Autodesk Inventor part; units mm, degrees
ref_plane "YZ Plane" through (0, 0, 0) normal (1, 0, 0) x (0, 1, 0)
ref_plane "XZ Plane" through (0, 0, 0) normal (0, 1, 0) x (-1, 0, 0)
ref_plane "XY Plane" through (0, 0, 0) normal (0, 0, 1) x (1, 0, 0)
sketch "Sketch1" plane through (0, 0, 0) normal (0, 0, 1) x (1, 0, 0)
  line L0 (-168.2745, 480.6024) -> (-113.8232, 480.6024)
  line L1 (-73.2956, 353.1342) -> (-73.2956, 2.8452)
  line L2 (-73.2956, 2.8452) -> (-375.9641, 2.8452)
  line L3 (-375.9641, 2.8452) -> (-375.9641, 41.7492)
  arc A0 (-375.9641, 41.7492) -> (-168.2745, 480.6024) centre (-397.1456, 320.3452) ccw
  line L4 (-168.2745, 480.6024) -> (-245.12, 590.3492) construction
  line L5 (-245.12, 590.3492) -> (-245.12, 480.6024) construction
  line L6 (-245.12, 480.6024) -> (-168.2745, 480.6024) construction
  line L7 (-117.7456, 320.3452) -> (-117.7456, 124.3972) construction
  line L8 (-397.1456, 40.9452) -> (-554.9899, 40.9452) construction
  arc A1 (-73.2956, 353.1342) -> (-113.8232, 480.6024) centre (-397.1456, 320.3452) ccw
  dimension "d4" = 279.4
  dimension "d6" = 55
  dimension "d17" = 44.45
  dimension "d22" = 38.1
extrude "Extrusion1" add sketch "Sketch1" along normal blind 1.5875
sketch "Sketch2" plane through (0, 0, 1.5875) normal (0, 0, 1) x (1, 0, 0)
  arc A0 (-375.9641, 41.7492) -> (-168.2745, 480.6024) centre (-397.1456, 320.3452) ccw
  arc A1 (-375.9641, 41.7492) -> (-168.2745, 480.6024) centre (-397.1456, 320.3452) ccw
  arc A2 (-375.603, 37.0004) -> (-164.3733, 483.3341) centre (-397.1456, 320.3452) ccw
  line L0 (-397.1456, 320.3452) -> (-164.3733, 483.3341)
  line L1 (-168.2745, 480.6024) -> (-164.3733, 483.3341)
  line L2 (-397.1456, 320.3452) -> (-375.603, 37.0004)
  line L3 (-375.603, 37.0004) -> (-375.9641, 41.7492)
  point P0 (0, 0)
  dimension "d21" = 4.7625
extrude "Extrusion2" add sketch "Sketch2" along normal blind 15.875 and the other way blind 19.05 contours A0 L0 A2 L2
fillet "Fillet1" radius 25.4 1 edges at (-113.8232, 480.6024, 0.7937)
properties part number "ShooterCurve" material "Aluminum-6061"
The model under review builds one solid part; all positions refer to its coordinate system, in mm. Give positions to 0.01 mm unless a question says otherwise; leave off trailing zeros. Loops run counter-clockwise (first coordinate to the right, second up) from the corner with the lowest first, then second, coordinate; pieces in that order, holes last. Notation, with made-up numbers: (39, 37.5) -> (95, 37.5) arc R28 cw to (95, 68.5) -> close; hole circle Ø10 at (54, -7). An arc over 180 degrees is marked (long way). Put each result on its own line as item: value. Start each with the question number.
1. We need section A-A on x = -144. State the section outline as (y, z) points.
2. Clearance check with flat-ended pins moving along their axes: P1, Ø1.5, axis at x = -270, z = 12, coming from the -Y side; P2, Ø1.3, axis at x = -143, z = 0.5, coming from the +Y side; P3, Ø1.5, axis at x = -249.5, z = 2.5, coming from the +Y side. State where each tip first meets the part, or that it passes through.
3. We need section C-C on x = -347. State the section outline as (y, z) points, then the cut area to 3 significant figures.
4. We need section B-B on y = 416.5. State the section outline as (x, z) points, then the cut area to 3 significant figures.
5. Wall thickness on probe 1 along Z at (x, y) = (-139.5, 141.5); probe 2 along Y at (x, z) = (-149.5, 10); probe 3 along Y at (x, z) = (-155.5, 10): over which ranges is each line inside the solid? List them lowest first.
6. Mouldability with a two-part tool opening along Y and no side actions: class faces 1 (the face through (-142.865, 204.562, -0.244)), 2 (the face through (-147, 137, 1.588)), 3 (the face through (-84.865, 412.187, 0.783)) as released by +Y, released by -Y, zero draft, split by the parting line, or undercut.
7. We need section D-D on z = 12.5. State the section outline as (x, y) points (1 decimal).
Determined:
1. outline: (2.85, 0) -> (191.25, 0) -> (191.25, -17.46) -> (202.1, -17.46) -> (202.1, 17.46) -> (191.25, 17.46) -> (191.25, 1.59) -> (2.85, 1.59) -> close; (438.59, -17.46) -> (449.44, -17.46) -> (449.44, 0) -> (480.6, 0) -> (480.6, 1.59) -> (449.44, 1.59) -> (449.44, 17.46) -> (438.59, 17.46) -> close
2. P1: y = 65.84
2. P2: y = 480.6
2. P3: y = 83.61
3. outline: (2.85, 0) -> (40.64, 0) -> (40.64, -17.46) -> (45.48, -17.46) -> (45.48, 17.46) -> (40.64, 17.46) -> (40.64, 1.59) -> (2.85, 1.59) -> close
3. area: 229 mm^2
4. outline: (-134.81, -17.46) -> (-129.75, -17.46) -> (-129.75, 0) -> (-86.17, 0) -> (-86.17, 1.59) -> (-129.75, 1.59) -> (-129.75, 17.46) -> (-134.81, 17.46) -> close
4. area: 246 mm^2
5. probe 1: 0 to 1.59
5. probe 2: 180.99 to 190.98, 449.71 to 459.7
5. probe 3: 170.83 to 180.09, 460.6 to 469.86
6. face 1: undercut
6. face 2: zero draft
6. face 3: released by +Y
7. outline: (-376, 41.7) -> (-375.6, 37) arc R284.2 ccw to (-164.4, 483.3) -> (-168.3, 480.6) arc R279.4 cw to start
